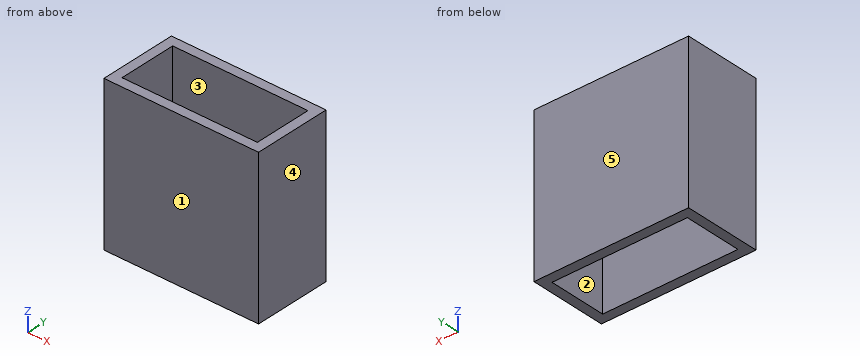
Autodesk Inventor part; units mm, degrees
ref_plane "Start Plane" through (0, 0, 0) normal (0, 0, 1) x (1, 0, 0)
ref_plane "End Plane" through (0, 0, 50.8) normal (0, 0, 1) x (1, 0, 0)
ref_plane "YZ Plane" through (0, 0, 0) normal (1, 0, 0) x (0, 1, 0)
ref_plane "Start Plane" through (0, 0, 0) normal (0, 0, 1) x (1, 0, 0)
ref_plane "End Plane" through (0, 0, 50.8) normal (0, 0, 1) x (1, 0, 0)
sketch "Sketch1" plane through (0, 0, 0) normal (0, 0, 1) x (1, 0, 0)
  line L0 (-25.4, 12.7) -> (25.4, 12.7)
  line L1 (25.4, 12.7) -> (25.4, -12.7)
  line L2 (25.4, -12.7) -> (-25.4, -12.7)
  line L3 (-25.4, -12.7) -> (-25.4, 12.7)
  line L4 (22.225, 9.525) -> (-22.225, 9.525)
  line L5 (-22.225, 9.525) -> (-22.225, -9.525)
  line L6 (-22.225, -9.525) -> (22.225, -9.525)
  line L7 (22.225, -9.525) -> (22.225, 9.525)
  point P0 (0, 0)
  point P1 (0, 12.7)
  point P2 (-25.4, 0)
  dimension "d0" = 50.8
  dimension "d1" = 25.4
  dimension "d2" = 3.175
extrude "Body" add sketch "Sketch1" along normal up to surface (50.8 mm away) from surface at 0
sketch "Sketch2" plane through (0, 0, 0) normal (0, 0, 1) x (1, 0, 0)
  line L0 (0, 0) -> (10, 0)
ref_plane "Work Plane3" through (0, 0, 0) normal (0, -1, 0) x (1, 0, 0)
sketch "Sketch3" plane through (0, 0, 0) normal (0, -1, 0) x (1, 0, 0)
  line L0 (-35.56, 0) -> (35.56, 0)
  line L1 (-35.56, 50.8) -> (35.56, 50.8)
  dimension "d10" = 50.8
equation "\"G_OFFSET_START\" = 0"
equation "\"G_OFFSET_END\" = 0"
equation "\"d6\" = length + G_OFFSET_END"
equation "\"G_L\" = d10"
properties part number "2x1x.125 Tube"
Read the model definition and answer for the solid it produces. Units are mm, in the model's axes. Face numbers are marked on the shaded views. A direction names the side the tool comes from. Round coordinates to 2 decimals unless told otherwise and drop trailing zeros. Loops run counter-clockwise (first coordinate to the right, second up) from the corner with the lowest first, then second, coordinate; pieces in that order, holes last. Notation, with made-up numbers: (-16, -23) - (28, -23) arc R34 cw to (28, 11) - close; hole circle Ø10 at (65, 46.25). An arc over 180 degrees is marked (long way). One line per question, with ' | ' between items. Start each with the question number.
Q1. Section B-B on y = -1.25 is taken. Give the vertices of the cut face in (x, z) (3 decimals), plus the area to 3 significant figures.
Q2. For a pull along Y with two mould halves and no side action, classify the marked faces 3, 4 and 5 as +Y half, -Y half, draft (parallel to the pull), parting line (faces both ways), or undercut.
Q3. Find the intervals of material crossed by L1, parallel to Y at x = 10.5, z = 29.5 (3 decimals); L2, parallel to X at y = 9, z = 17.5 (3 decimals), in increasing order.
Q4. For the marked faces 1 and 2, determine the directions among +Z, -Z, +X, -X, +Y, -Y from which every point of the face is accessible in a straight line to the end or side of a thin tool.
Q5. Section C-C on x = 8 is taken. Give the vertices of the cut face in (y, z) (3 decimals), plus the area to 3 significant figures.
Q6. Section A-A on z = 14 is taken. Give the vertices of the cut face in (x, y) (3 decimals).
Established:
1) outline: (-25.4, 0) - (-22.225, 0) - (-22.225, 50.8) - (-25.4, 50.8) - close; (22.225, 0) - (25.4, 0) - (25.4, 50.8) - (22.225, 50.8) - close | area: 323 mm²
2) face 3: undercut | face 4: draft | face 5: +Y half
3) L1: -12.7 to -9.525, 9.525 to 12.7 | L2: -25.4 to -22.225, 22.225 to 25.4
4) face 1: +Z, -Z, +X, -X, -Y | face 2: +Z, -Z
5) outline: (-12.7, 0) - (-9.525, 0) - (-9.525, 50.8) - (-12.7, 50.8) - close; (9.525, 0) - (12.7, 0) - (12.7, 50.8) - (9.525, 50.8) - close | area: 323 mm²
6) outline: (-25.4, -12.7) - (25.4, -12.7) - (25.4, 12.7) - (-25.4, 12.7) - close; hole (-22.225, -9.525) - (22.225, -9.525) - (22.225, 9.525) - (-22.225, 9.525) - close
